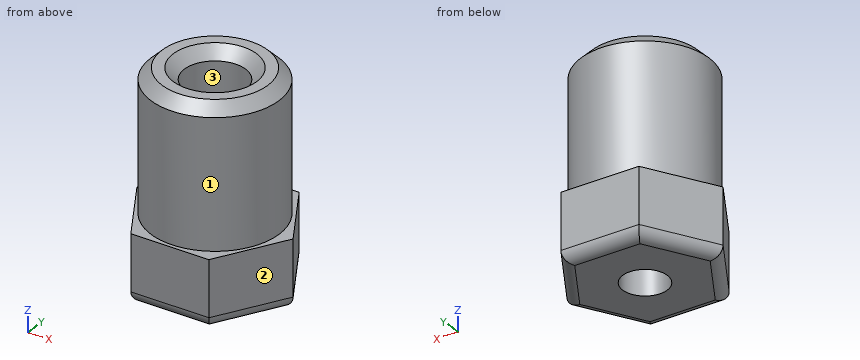
```python
from build123d import *

# Parameters (mm, degrees)
PAD_DEPTH     = 6
SKETCH001_R   = 5.75
SKETCH001_R_2 = 2.75
PAD001_DEPTH  = 12.5
CHAMFER_SIZE  = 1
FILLET_R      = 1
SKETCH002_R   = 2
POCKET_DEPTH  = 18.501


with BuildPart() as part:
    # Sketch → Pad (new body)
    with BuildSketch(Plane.XY):
        Polygon((3.5, -6.062178), (7, 0), (3.5, 6.062178), (-3.5, 6.062178), (-7, 0), (-3.5, -6.062178), align=None)
    extrude(amount=PAD_DEPTH)

    # Sketch001 → Pad001 (join)
    with BuildSketch(Plane.XY.offset(6)):
        Circle(SKETCH001_R)
        Circle(SKETCH001_R_2, mode=Mode.SUBTRACT)
    extrude(amount=PAD001_DEPTH)

    # Chamfer
    chamfer_edges = [part.edges().sort_by_distance(p)[0] for p in [
        (-2.75, 0, 18.5),
        (-5.75, 0, 18.5),
    ]]
    chamfer(chamfer_edges, length=CHAMFER_SIZE)

    # Fillet
    fillet_edges = [part.edges().sort_by_distance(p)[0] for p in [
        (5.25, 3.031089, 0),
        (5.25, -3.031089, 0),
        (0, -6.062178, 0),
        (-5.25, -3.031089, 0),
        (-5.25, 3.031089, 0),
        (0, 6.062178, 0),
    ]]
    fillet(fillet_edges, radius=FILLET_R)

    # Sketch002 → Pocket (cut, through all)
    with BuildSketch(Plane.XY):
        Circle(SKETCH002_R)
    extrude(amount=POCKET_DEPTH, mode=Mode.SUBTRACT)


solid = part.part
```
Build history of the part. All positions in model axes, mm. Face numbers are marked on the shaded views. Give positions to 0.01 mm unless a question says otherwise; leave off trailing zeros. Loops run counter-clockwise (first coordinate to the right, second up) from the corner with the lowest first, then second, coordinate; pieces in that order, holes last.
1) Probe line 1 along Y through (x, z) = (0, 12); line 2 along Y through (x, z) = (0, 4.5); line 3 along X through (y, z) = (-1, 3.75). List the from-to ranges inside material, lowest first.
Values follow:
line 1: y = -5.75 to -2.75, 2.75 to 5.75
line 2: y = -6.06 to -2, 2 to 6.06
line 3: x = -6.42 to -1.73, 1.73 to 6.42
2) Band-saw the part on C-C on z = 10.75. List the corners of the cut face in (x, y), then the cut area to 3 significant figures.
Values follow:
outline: circle Ø11.5 at (0, 0); hole circle Ø5.5 at (0, 0)
area: 80.1 mm2
3) Band-saw the part on B-B on x = 0. List the corners of the cut face in (y, z).
Values follow:
outline: (-6.06, 1) arc R1 ccw to (-5.06, 0) - (-2, 0) - (-2, 6) - (-2.75, 6) - (-2.75, 17.5) - (-3.75, 18.5) - (-4.75, 18.5) - (-5.75, 17.5) - (-5.75, 6) - (-6.06, 6) - close; (2, 0) - (5.06, 0) arc R1 ccw to (6.06, 1) - (6.06, 6) - (5.75, 6) - (5.75, 17.5) - (4.75, 18.5) - (3.75, 18.5) - (2.75, 17.5) - (2.75, 6) - (2, 6) - close
4) Two-plate mould, pull along Y, no slides. Class the marked faces 1, 2 and 3: released by +Y, released by -Y, zero draft, split by the parting line, or undercut.
Values follow:
face 1: split by the parting line
face 2: released by -Y
face 3: undercut
5) Drop flat-ended pins along their axis: P1, Ø5, axis at y = 3.5, z = 2.5, coming from the +X side; P2, Ø6, axis at x = 3, z = 15, coming from the +Y side; P3, Ø6, axis at y = -4.5, z = 9.5, coming from the -X side. Give the stop position or say it passes through.
Values follow:
P1: stops at x = 6.42
P2: stops at y = 5.75
P3: stops at x = -5.55
6) Band-saw the part on A-A on z = 4.25. List the corners of the cut face in (x, y).
Values follow:
outline: (-7, 0) - (-3.5, -6.06) - (3.5, -6.06) - (7, 0) - (3.5, 6.06) - (-3.5, 6.06) - close; hole circle Ø4 at (0, 0)
